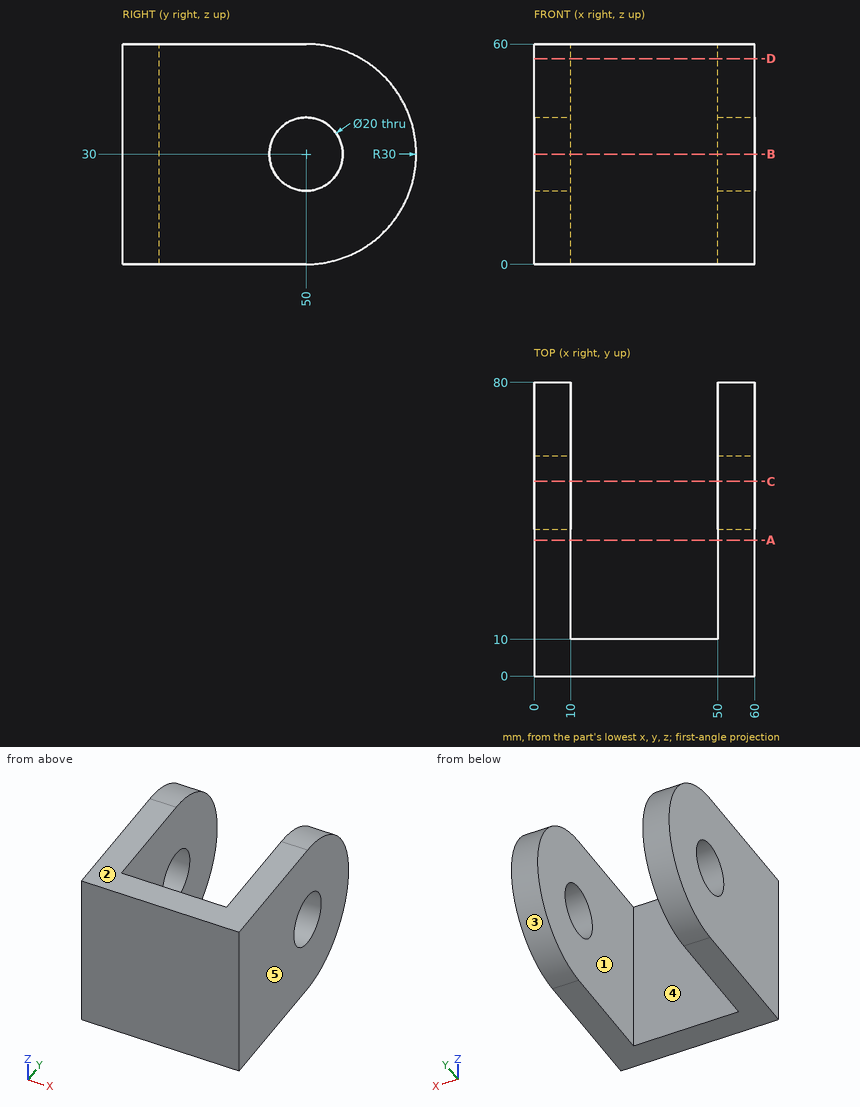
Job drawing, mm, ordinate dimensions from the low corner. One solid piece. A direction names the side the tool comes from. Give positions to 0.01 mm unless a question says otherwise; leave off trailing zeros. Order: outer loops, then holes, each group sorted by start corner. A loop starts at its lowest first (then second) coordinate and runs counter-clockwise, first axis right, second up. Notation, with made-up numbers: (-26, -3) - (-22, -3) arc R21 cw to (-22, 7) - close; hole circle Ø4 at (43, 5.25). An arc over 180 degrees is marked (long way). Answer in a Markdown table with one row per item.
1. Probe probe 1 along X at (y, z) = (32, 46); probe 2 along Z at (x, y) = (4.5, 50); probe 3 along Y at (x, z) = (6, 30). List the from-to ranges inside material, lowest first. Write a range as [from, to].
Data:
| item | result |
|---|---|
| probe 1 | x = [0, 10], [50, 60] |
| probe 2 | z = [0, 20], [40, 60] |
| probe 3 | y = [0, 40], [60, 80] |
2. Flat gauge pin, fed straight in: pin 1 (4 mm diameter, centred on x = 13, z = 10.5, fed in from +Y). Where does the tip first touch, or does it go through?
Data:
| item | result |
|---|---|
| pin 1 | stops at y = 10 |
3. Saw through at C-C, the plane y = 53. Give the cut face in (x, z), plus the area to 3 significant figures.
Data:
| item | result |
|---|---|
| outline | (0, 0.15) - (10, 0.15) - (10, 20.46) - (0, 20.46) - close; (0, 39.54) - (10, 39.54) - (10, 59.85) - (0, 59.85) - close; (50, 0.15) - (60, 0.15) - (60, 20.46) - (50, 20.46) - close; (50, 39.54) - (60, 39.54) - (60, 59.85) - (50, 59.85) - close |
| area | 812 mm² |
4. Saw through at D-D, the plane z = 56. Give the cut face in (x, y), plus the area to 3 significant figures.
Data:
| item | result |
|---|---|
| outline | (0, 0) - (60, 0) - (60, 64.97) - (50, 64.97) - (50, 10) - (10, 10) - (10, 64.97) - (0, 64.97) - close |
| area | 1,700 mm² |
5. Saw through at B-B, the plane z = 30. Give the cut face in (x, y).
Data:
| item | result |
|---|---|
| outline | (0, 0) - (60, 0) - (60, 40) - (50, 40) - (50, 10) - (10, 10) - (10, 40) - (0, 40) - close; (0, 60) - (10, 60) - (10, 80) - (0, 80) - close; (50, 60) - (60, 60) - (60, 80) - (50, 80) - close |
6. Pull direction X, two halves, no side cores. Call the marked faces 3, 4 and 5: pulls with the +X half, pulls with the -X half, needs draft (parallel to the pull), parting line crosses it, or undercut.
Data:
| item | result |
|---|---|
| face 3 | needs draft |
| face 4 | undercut |
| face 5 | pulls with the +X half |
7. Saw through at A-A, the plane y = 37. Give the cut face in (x, z).
Data:
| item | result |
|---|---|
| outline | (0, 0) - (10, 0) - (10, 60) - (0, 60) - close; (50, 0) - (60, 0) - (60, 60) - (50, 60) - close |
8. Tool access for the marked faces 1 and 2: list every direction of +Z, -Z, +X, -X, +Y, -Y with a clear straight run to the whole face (end or side of a thin tool).
Data:
| item | result |
|---|---|
| face 1 | +Z, -Z, +Y |
| face 2 | +Z, +X, -X, +Y, -Y |
